Input: part model. Units: mm. Frame: model coordinates. Face numbers are marked on the shaded views. Coordinates: 2 decimals unless noted, no trailing zeros. Write each loop counter-clockwise with the first axis right and the second up, starting at its lowest first coordinate (ties: lowest second). Pieces come first, ordered by that corner, then holes.
1) Section query A-A (y = 116.5). Output: boundary loops of the cut face in (x, z), then the cut area to 3 significant figures.
2) Section query B-B (z = -62.5). Output: boundary loops of the cut face in (x, y), then the cut area to 3 significant figures.
3) Line query: L1, parallel to Z at x = 0.75, y = 73.5; L2, parallel to X at y = 77, z = -192; L3, parallel to Z at x = 301.65, y = 151.5. Output: solid intervals per line, ascending.
4) Pin query (flat end, axial travel): pin 1 Ø1.2 at (x, z) = (301, -187.5) entering from -Y; pin 2 Ø2.5 at (y, z) = (14.5, -197) entering from -X; pin 3 Ø2 at (x, z) = (195.5, -135) entering from +Y. Return the tip coordinate at first contact, or that it passes through.
5) Draft query along X for the marked faces 1, 2, 3 and 4. Return one class per face: pulls with the +X half, pulls with the -X half, needs draft (parallel to the pull), parting line crosses it, or undercut.
6) Section query C-C (x = 195). Output: boundary loops of the cut face in (y, z).
from build123d import *

# Parameters (mm, degrees)
SKETCH_1_W                         = 302
SKETCH_1_H                         = 207
SM_BASE_FLANGE_1_DEPTH             = 1.5
SM_EDGE_FLANGE_1_STRIP_W           = 7.4732
SM_EDGE_FLANGE_1_STRIP_H           = 1.5
SM_EDGE_FLANGE_1_STRIP_CUT_DEPTH   = 207
SM_EDGE_FLANGE_1_STRIP_2_W         = 7.4732
SM_EDGE_FLANGE_1_STRIP_2_H         = 1.5
SM_EDGE_FLANGE_1_STRIP_CUT_2_DEPTH = 207
SM_EDGE_FLANGE_1_DEPTH             = 207
SM_EDGE_FLANGE_1_BEND_DEPTH        = 207
CUT_EXTRUDE_1_REACH                = 406.308
SKETCH_12_W                        = 4
SKETCH_12_H                        = 60
CUT_EXTRUDE_2_REACH                = 406.308
SKETCH_13_R                        = 2
CUT_EXTRUDE_3_REACH                = 406.308
SKETCH_14_R                        = 2
CUT_EXTRUDE_4_REACH                = 406.308
SKETCH_15_R                        = 2


# Sheet-metal steps are written as plain solids
with BuildPart() as part:
    # Sketch 1 → Базовая кромка1 (new body)
    with BuildSketch(Plane(origin=(0, 0, 0), x_dir=(1, 0, 0), z_dir=(0, 1, 0))):
        with Locations((151, 103.5)):
            Rectangle(SKETCH_1_W, SKETCH_1_H)
    extrude(amount=-SM_BASE_FLANGE_1_DEPTH)

    # Ребро-кромка1 strip (across the edge) → Ребро-кромка1 strip cut (cut)
    with BuildSketch(Plane.XY.offset(-207)):
        with Locations((-1.5, -0.75)):
            Rectangle(SM_EDGE_FLANGE_1_STRIP_W, SM_EDGE_FLANGE_1_STRIP_H)
    extrude(amount=SM_EDGE_FLANGE_1_STRIP_CUT_DEPTH, mode=Mode.SUBTRACT)

    # Ребро-кромка1 strip 2 (across the edge) → Ребро-кромка1 strip cut 2 (cut)
    with BuildSketch(Plane(origin=(302, 0, 0), x_dir=(-1, 0, 0), z_dir=(0, 0, -1))):
        with Locations((-1.5, -0.75)):
            Rectangle(SM_EDGE_FLANGE_1_STRIP_2_W, SM_EDGE_FLANGE_1_STRIP_2_H)
    extrude(amount=SM_EDGE_FLANGE_1_STRIP_CUT_2_DEPTH, mode=Mode.SUBTRACT)

    # Ребро-кромка1 section (across the edge) → Ребро-кромка1 (add)
    with BuildSketch(Plane.XY.offset(-207)):
        with BuildLine():
            Line((0, 0.7366), (0, 171.5))
            Line((0, 171.5), (1.5, 171.5))
            Line((1.5, 171.5), (1.5, 0.7366))
            ThreePointArc((1.5, 0.7366), (1.715745145, 0.215745145), (2.2366, 0))
            Line((2.2366, 0), (2.2366, -1.5))
            ThreePointArc((2.2366, -1.5), (0.655084973, -0.844915027), (0, 0.7366))
        make_face()
    extrude(amount=SM_EDGE_FLANGE_1_DEPTH)

    # Ребро-кромка1 section 2 (across the edge) → Ребро-кромка1 bend (add)
    with BuildSketch(Plane(origin=(302, 0, 0), x_dir=(-1, 0, 0), z_dir=(0, 0, -1))):
        with BuildLine():
            Line((0, 0.7366), (0, 171.5))
            Line((0, 171.5), (1.5, 171.5))
            Line((1.5, 171.5), (1.5, 0.7366))
            ThreePointArc((1.5, 0.7366), (1.715745145, 0.215745145), (2.2366, 0))
            Line((2.2366, 0), (2.2366, -1.5))
            ThreePointArc((2.2366, -1.5), (0.655084973, -0.844915027), (0, 0.7366))
        make_face()
    extrude(amount=SM_EDGE_FLANGE_1_BEND_DEPTH)

    # Эскиз12 → Вырез-Вытянуть1 (cut, up to next)
    with BuildSketch(Plane(origin=(302, 0, 0), x_dir=(0, 0, -1), z_dir=(1, 0, 0)), mode=Mode.PRIVATE) as cut_extrude_1_sk1:
        with Locations((187, 76.5)):
            Rectangle(SKETCH_12_W, SKETCH_12_H)
    cut_extrude_1_tool1 = extrude(cut_extrude_1_sk1.sketch, amount=-CUT_EXTRUDE_1_REACH, mode=Mode.PRIVATE) & part.part
    # Эскиз12 → Вырез-Вытянуть1 (cut, up to next)
    with BuildSketch(Plane(origin=(302, 0, 0), x_dir=(0, 0, -1), z_dir=(1, 0, 0)), mode=Mode.PRIVATE) as cut_extrude_1_sk2:
        with Locations((20, 76.5)):
            Rectangle(SKETCH_12_W, SKETCH_12_H)
    cut_extrude_1_tool2 = extrude(cut_extrude_1_sk2.sketch, amount=-CUT_EXTRUDE_1_REACH, mode=Mode.PRIVATE) & part.part
    add(cut_extrude_1_tool1.solids().sort_by_distance((302, 76.5, -187))[0], mode=Mode.SUBTRACT)
    add(cut_extrude_1_tool2.solids().sort_by_distance((302, 76.5, -20))[0], mode=Mode.SUBTRACT)

    # Эскиз13 → Вырез-Вытянуть2 (cut, up to next)
    with BuildSketch(Plane.ZY, mode=Mode.PRIVATE) as cut_extrude_2_sk1:
        with Locations(Location((-197, 88.5, 0), (0, 0, 270))):
            Circle(SKETCH_13_R)
    cut_extrude_2_tool1 = extrude(cut_extrude_2_sk1.sketch, amount=-CUT_EXTRUDE_2_REACH, mode=Mode.PRIVATE) & part.part
    # Эскиз13 → Вырез-Вытянуть2 (cut, up to next)
    with BuildSketch(Plane.ZY, mode=Mode.PRIVATE) as cut_extrude_2_sk2:
        with Locations(Location((-197, 73.5, 0), (0, 0, 270))):
            Circle(SKETCH_13_R)
    cut_extrude_2_tool2 = extrude(cut_extrude_2_sk2.sketch, amount=-CUT_EXTRUDE_2_REACH, mode=Mode.PRIVATE) & part.part
    # Эскиз13 → Вырез-Вытянуть2 (cut, up to next)
    with BuildSketch(Plane.ZY, mode=Mode.PRIVATE) as cut_extrude_2_sk3:
        with Locations(Location((-197, 29.5, 0), (0, 0, 270))):
            Circle(SKETCH_13_R)
    cut_extrude_2_tool3 = extrude(cut_extrude_2_sk3.sketch, amount=-CUT_EXTRUDE_2_REACH, mode=Mode.PRIVATE) & part.part
    # Эскиз13 → Вырез-Вытянуть2 (cut, up to next)
    with BuildSketch(Plane.ZY, mode=Mode.PRIVATE) as cut_extrude_2_sk4:
        with Locations(Location((-197, 14.5, 0), (0, 0, 270))):
            Circle(SKETCH_13_R)
    cut_extrude_2_tool4 = extrude(cut_extrude_2_sk4.sketch, amount=-CUT_EXTRUDE_2_REACH, mode=Mode.PRIVATE) & part.part
    # Эскиз13 → Вырез-Вытянуть2 (cut, up to next)
    with BuildSketch(Plane.ZY, mode=Mode.PRIVATE) as cut_extrude_2_sk5:
        with Locations(Location((-10, 14.5, 0), (0, 0, 270))):
            Circle(SKETCH_13_R)
    cut_extrude_2_tool5 = extrude(cut_extrude_2_sk5.sketch, amount=-CUT_EXTRUDE_2_REACH, mode=Mode.PRIVATE) & part.part
    # Эскиз13 → Вырез-Вытянуть2 (cut, up to next)
    with BuildSketch(Plane.ZY, mode=Mode.PRIVATE) as cut_extrude_2_sk6:
        with Locations(Location((-10, 29.5, 0), (0, 0, 270))):
            Circle(SKETCH_13_R)
    cut_extrude_2_tool6 = extrude(cut_extrude_2_sk6.sketch, amount=-CUT_EXTRUDE_2_REACH, mode=Mode.PRIVATE) & part.part
    # Эскиз13 → Вырез-Вытянуть2 (cut, up to next)
    with BuildSketch(Plane.ZY, mode=Mode.PRIVATE) as cut_extrude_2_sk7:
        with Locations(Location((-10, 73.5, 0), (0, 0, 270))):
            Circle(SKETCH_13_R)
    cut_extrude_2_tool7 = extrude(cut_extrude_2_sk7.sketch, amount=-CUT_EXTRUDE_2_REACH, mode=Mode.PRIVATE) & part.part
    # Эскиз13 → Вырез-Вытянуть2 (cut, up to next)
    with BuildSketch(Plane.ZY, mode=Mode.PRIVATE) as cut_extrude_2_sk8:
        with Locations(Location((-10, 88.5, 0), (0, 0, 270))):
            Circle(SKETCH_13_R)
    cut_extrude_2_tool8 = extrude(cut_extrude_2_sk8.sketch, amount=-CUT_EXTRUDE_2_REACH, mode=Mode.PRIVATE) & part.part
    add(cut_extrude_2_tool1.solids().sort_by_distance((0, 88.5, -197))[0], mode=Mode.SUBTRACT)
    add(cut_extrude_2_tool2.solids().sort_by_distance((0, 73.5, -197))[0], mode=Mode.SUBTRACT)
    add(cut_extrude_2_tool3.solids().sort_by_distance((0, 29.5, -197))[0], mode=Mode.SUBTRACT)
    add(cut_extrude_2_tool4.solids().sort_by_distance((0, 14.5, -197))[0], mode=Mode.SUBTRACT)
    add(cut_extrude_2_tool5.solids().sort_by_distance((0, 14.5, -10))[0], mode=Mode.SUBTRACT)
    add(cut_extrude_2_tool6.solids().sort_by_distance((0, 29.5, -10))[0], mode=Mode.SUBTRACT)
    add(cut_extrude_2_tool7.solids().sort_by_distance((0, 73.5, -10))[0], mode=Mode.SUBTRACT)
    add(cut_extrude_2_tool8.solids().sort_by_distance((0, 88.5, -10))[0], mode=Mode.SUBTRACT)

    # Эскиз14 → Вырез-Вытянуть3 (cut, up to next)
    with BuildSketch(Plane.ZY, mode=Mode.PRIVATE) as cut_extrude_3_sk1:
        with Locations(Location((-192, 151.5, 0), (0, 0, 270))):
            Circle(SKETCH_14_R)
    cut_extrude_3_tool1 = extrude(cut_extrude_3_sk1.sketch, amount=-CUT_EXTRUDE_3_REACH, mode=Mode.PRIVATE) & part.part
    # Эскиз14 → Вырез-Вытянуть3 (cut, up to next)
    with BuildSketch(Plane.ZY, mode=Mode.PRIVATE) as cut_extrude_3_sk2:
        with Locations(Location((-15, 151.5, 0), (0, 0, 270))):
            Circle(SKETCH_14_R)
    cut_extrude_3_tool2 = extrude(cut_extrude_3_sk2.sketch, amount=-CUT_EXTRUDE_3_REACH, mode=Mode.PRIVATE) & part.part
    # Эскиз14 → Вырез-Вытянуть3 (cut, up to next)
    with BuildSketch(Plane.ZY, mode=Mode.PRIVATE) as cut_extrude_3_sk3:
        with Locations(Location((-15, 51.5, 0), (0, 0, 270))):
            Circle(SKETCH_14_R)
    cut_extrude_3_tool3 = extrude(cut_extrude_3_sk3.sketch, amount=-CUT_EXTRUDE_3_REACH, mode=Mode.PRIVATE) & part.part
    # Эскиз14 → Вырез-Вытянуть3 (cut, up to next)
    with BuildSketch(Plane.ZY, mode=Mode.PRIVATE) as cut_extrude_3_sk4:
        with Locations(Location((-192, 51.5, 0), (0, 0, 270))):
            Circle(SKETCH_14_R)
    cut_extrude_3_tool4 = extrude(cut_extrude_3_sk4.sketch, amount=-CUT_EXTRUDE_3_REACH, mode=Mode.PRIVATE) & part.part
    add(cut_extrude_3_tool1.solids().sort_by_distance((0, 151.5, -192))[0], mode=Mode.SUBTRACT)
    add(cut_extrude_3_tool2.solids().sort_by_distance((0, 151.5, -15))[0], mode=Mode.SUBTRACT)
    add(cut_extrude_3_tool3.solids().sort_by_distance((0, 51.5, -15))[0], mode=Mode.SUBTRACT)
    add(cut_extrude_3_tool4.solids().sort_by_distance((0, 51.5, -192))[0], mode=Mode.SUBTRACT)

    # Эскиз15 → Вырез-Вытянуть4 (cut, up to next)
    with BuildSketch(Plane(origin=(302, 0, 0), x_dir=(0, 0, -1), z_dir=(1, 0, 0)), mode=Mode.PRIVATE) as cut_extrude_4_sk1:
        with Locations(Location((15, 151.5, 0), (0, 0, 270))):
            Circle(SKETCH_15_R)
    cut_extrude_4_tool1 = extrude(cut_extrude_4_sk1.sketch, amount=-CUT_EXTRUDE_4_REACH, mode=Mode.PRIVATE) & part.part
    # Эскиз15 → Вырез-Вытянуть4 (cut, up to next)
    with BuildSketch(Plane(origin=(302, 0, 0), x_dir=(0, 0, -1), z_dir=(1, 0, 0)), mode=Mode.PRIVATE) as cut_extrude_4_sk2:
        with Locations(Location((192, 151.5, 0), (0, 0, 270))):
            Circle(SKETCH_15_R)
    cut_extrude_4_tool2 = extrude(cut_extrude_4_sk2.sketch, amount=-CUT_EXTRUDE_4_REACH, mode=Mode.PRIVATE) & part.part
    # Эскиз15 → Вырез-Вытянуть4 (cut, up to next)
    with BuildSketch(Plane(origin=(302, 0, 0), x_dir=(0, 0, -1), z_dir=(1, 0, 0)), mode=Mode.PRIVATE) as cut_extrude_4_sk3:
        with Locations(Location((15, 18.5, 0), (0, 0, 90))):
            Circle(SKETCH_15_R)
    cut_extrude_4_tool3 = extrude(cut_extrude_4_sk3.sketch, amount=-CUT_EXTRUDE_4_REACH, mode=Mode.PRIVATE) & part.part
    # Эскиз15 → Вырез-Вытянуть4 (cut, up to next)
    with BuildSketch(Plane(origin=(302, 0, 0), x_dir=(0, 0, -1), z_dir=(1, 0, 0)), mode=Mode.PRIVATE) as cut_extrude_4_sk4:
        with Locations(Location((192, 18.5, 0), (0, 0, 90))):
            Circle(SKETCH_15_R)
    cut_extrude_4_tool4 = extrude(cut_extrude_4_sk4.sketch, amount=-CUT_EXTRUDE_4_REACH, mode=Mode.PRIVATE) & part.part
    add(cut_extrude_4_tool1.solids().sort_by_distance((302, 151.5, -15))[0], mode=Mode.SUBTRACT)
    add(cut_extrude_4_tool2.solids().sort_by_distance((302, 151.5, -192))[0], mode=Mode.SUBTRACT)
    add(cut_extrude_4_tool3.solids().sort_by_distance((302, 18.5, -15))[0], mode=Mode.SUBTRACT)
    add(cut_extrude_4_tool4.solids().sort_by_distance((302, 18.5, -192))[0], mode=Mode.SUBTRACT)


solid = part.part
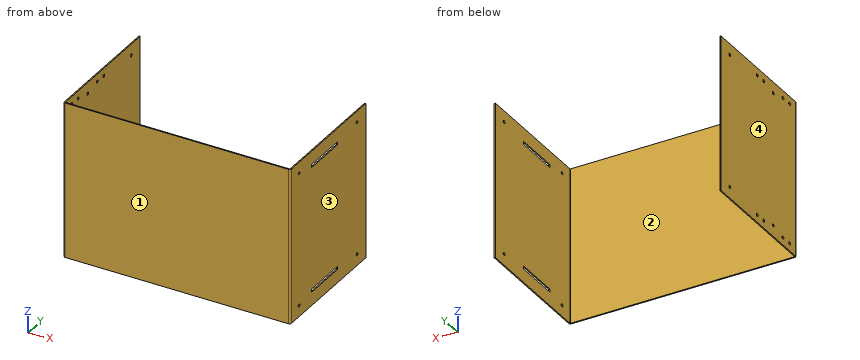
Answer:
1. outline: (0, -207) - (1.5, -207) - (1.5, 0) - (0, 0) - close; (300.5, -207) - (302, -207) - (302, 0) - (300.5, 0) - close
1. area: 621 mm2
2. outline: (0, 0.74) arc R2.24 ccw to (2.24, -1.5) - (299.76, -1.5) arc R2.24 ccw to (302, 0.74) - (302, 171.5) - (300.5, 171.5) - (300.5, 0.74) arc R0.74 cw to (299.76, 0) - (2.24, 0) arc R0.74 cw to (1.5, 0.74) - (1.5, 171.5) - (0, 171.5) - close
2. area: 966 mm2
3. L1: z = -207 to -199, -195 to -12, -8 to 0
3. L2: x = 0 to 1.5, 300.5 to 302
3. L3: z = -207 to -194, -190 to -17, -13 to 0
4. pin 1: stops at y = -1.41
4. pin 2: stops at x = 300.5
4. pin 3: stops at y = 0
5. face 1: needs draft
5. face 2: undercut
5. face 3: pulls with the +X half
5. face 4: pulls with the -X half
6. outline: (-1.5, -207) - (0, -207) - (0, 0) - (-1.5, 0) - close
